from build123d import *

# Parameters (mm, degrees)
SKETCH2_R           = 13.65
BOSS_EXTRUDE1_DEPTH = 8
SKETCH3_W           = 30
SKETCH3_H           = 34.126910457
BOSS_EXTRUDE2_DEPTH = 8
FILLET1_R           = 1
SKETCH5_R           = 2
CUT_EXTRUDE2_DEPTH  = 63.689475997


with BuildPart() as part:
    # Sketch2 → Boss-Extrude1 (new body)
    with BuildSketch(Plane.XY):
        with BuildLine():
            Line((22.912878475, 16.112283523), (-17.087121525, 16.112283523))
            Line((-17.087121525, 16.112283523), (-17.087121525, -17.887716477))
            Line((-17.087121525, -17.887716477), (22.912878475, -17.887716477))
            ThreePointArc((22.912878475, -17.887716477), (39.912878475, -0.887716477), (22.912878475, 16.112283523))
        make_face()
        with Locations((22.912878475, -0.887716477)):
            Circle(SKETCH2_R, mode=Mode.SUBTRACT)
    extrude(amount=BOSS_EXTRUDE1_DEPTH)

    # Sketch3 → Boss-Extrude2 (add)
    with BuildSketch(Plane.ZY.offset(17.087121525)):
        with Locations((4, -0.824261249)):
            Rectangle(SKETCH3_W, SKETCH3_H)
    extrude(amount=-BOSS_EXTRUDE2_DEPTH)

    # Fillet1
    fillet1_edges = [part.edges().sort_by_distance(p)[0] for p in [
        (-9.087121525, -0.887716477, 8),
        (-9.087121525, -0.887716477, 0),
    ]]
    fillet(fillet1_edges, radius=FILLET1_R)

    # Sketch5 → Cut-Extrude2 (cut, through all)
    with BuildSketch(Plane.ZY.offset(17.087121525)):
        with Locations(Location((-6, -0.824261249, 0), (0, 0, 270))):
            Circle(SKETCH5_R)
        with Locations(Location((14, -0.824261249, 0), (0, 0, 270))):
            Circle(SKETCH5_R)
    extrude(amount=-CUT_EXTRUDE2_DEPTH, mode=Mode.SUBTRACT)


solid = part.part
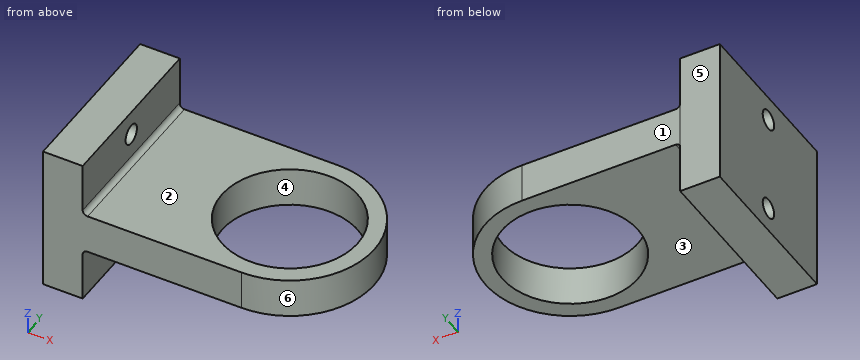
Read the model definition and answer for the solid it produces. Units are mm, in the model's axes. Face numbers are marked on the shaded views. A direction names the side the tool comes from. Round coordinates to 2 decimals unless told otherwise and drop trailing zeros. Order: outer loops, then holes, each group sorted by start corner. A loop starts at its lowest first (then second) coordinate and runs counter-clockwise, first axis right, second up.
1) For the marked faces 1, 2 and 3, determine the directions among +Z, -Z, +X, -X, +Y, -Y from which every point of the face is accessible in a straight line to the end or side of a thin tool.
2) Flat-ended cylindrical pins translate along their axes: pin 1 (5 mm diameter, centred on x = 2, y = 9, fed in from +Z); pin 2 (6 mm diameter, centred on x = -3, z = 3, fed in from +Y). Find the tip coordinate at first contact, or state that the pin passes through.
3) The mould has two halves that part along X. Classify the marked faces 4, 5 and 6: released by +X, released by -X, zero draft, split by the parting line, or undercut.
4) The part is cut by section D-D on x = 31.5. Write down the section's boundary in (y, z).
5) The part is cut by section B-B on x = -13. Write down the section's boundary in (y, z).
6) The part is cut by section C-C on y = -12. Write down the section's boundary in (x, z), plus the area to 3 significant figures.
7) The part is cut by section A-A on z = 14. Write down the section's boundary in (x, y).
8) Straight lines are drawn through the part: L1, parallel to Z at x = -5, y = 12; L2, parallel to X at y = -15.5, z = 13.5; L3, parallel to Y at x = 3.5, z = 4. For each, find the intervals that lie inside material, in ascending order.
Resolved:
1. face 1: +Z, -Z, +X, +Y
1. face 2: +Z, +X, +Y, -Y
1. face 3: -Z, +X, +Y, -Y
2. pin 1: stops at z = 8
2. pin 2: stops at y = 16.11
3. face 4: undercut
3. face 5: zero draft
3. face 6: released by +X
4. outline: (-15.56, 0) - (-11.5, 0) - (-11.5, 8) - (-15.56, 8) - close; (9.72, 0) - (13.78, 0) - (13.78, 8) - (9.72, 8) - close
5. outline: (-17.89, -11) - (16.24, -11) - (16.24, 19) - (-17.89, 19) - close; hole circle Ø4 at (-0.82, -6); hole circle Ø4 at (-0.82, 14)
6. outline: (-17.09, -11) - (-9.09, -11) - (-9.09, -1) arc R1 cw to (-8.09, 0) - (14.99, 0) - (14.99, 8) - (-8.09, 8) arc R1 cw to (-9.09, 9) - (-9.09, 19) - (-17.09, 19) - close; (30.84, 0) - (35.78, 0) - (35.78, 8) - (30.84, 8) - close
6. area: 473 mm2
7. outline: (-17.09, -17.89) - (-9.09, -17.89) - (-9.09, -2.82) - (-17.09, -2.82) - close; (-17.09, 1.18) - (-9.09, 1.18) - (-9.09, 16.24) - (-17.09, 16.24) - close
8. L1: z = 0 to 8
8. L2: x = -17.09 to -9.09
8. L3: y = -17.89 to 16.11
